Here's how the part is built. I have some questions about the finished solid (model axes, mm). A direction names the side the tool comes from. Round coordinates to 2 decimals unless told otherwise and drop trailing zeros. Loops run counter-clockwise (first coordinate to the right, second up) from the corner with the lowest first, then second, coordinate; pieces in that order, holes last. Notation, with made-up numbers: M 75,81.5 L 113,81.5 A24 ccw 113,115.5 Z; hole C 65.25,-34.5 d1. An arc over 180 degrees is marked long. Answer as CSV lines item,"result".
Autodesk Inventor part; units mm, degrees
ref_plane "YZ Plane" through (0, 0, 0) normal (1, 0, 0) x (0, 1, 0)
ref_plane "XZ Plane" through (0, 0, 0) normal (0, 1, 0) x (-1, 0, 0)
ref_plane "XY Plane" through (0, 0, 0) normal (0, 0, 1) x (1, 0, 0)
sketch "Sketch1" plane through (0, 0, 0) normal (0, 1, 0) x (-1, 0, 0)
  line L0 (27.5, -0.0615) -> (27.5, 89.9385)
  line L1 (-32.5, 89.9385) -> (-32.5, -0.0615)
  line L2 (-32.5, -0.0615) -> (-2.5, -0.0615)
  line L3 (-2.5, -0.0615) -> (-2.5, 89.9385) construction
  line L4 (-32.5, 44.9385) -> (-2.5, 44.9385) construction
  line L5 (-32.5, 89.9385) -> (27.5, 89.9385)
  line L6 (-21, 89.9385) -> (-9, 89.9385)
  line L7 (-9, 89.9385) -> (-9, 95.9385)
  line L8 (-9, 95.9385) -> (-21, 95.9385)
  line L9 (-21, 95.9385) -> (-21, 89.9385)
  line L10 (16, 89.9385) -> (4, 89.9385)
  line L11 (4, 89.9385) -> (4, 95.9385)
  line L12 (4, 95.9385) -> (16, 95.9385)
  line L13 (16, 95.9385) -> (16, 89.9385)
  line L14 (-2.5, 44.9385) -> (27.5, 44.9385) construction
  line L15 (-2.5, -0.0615) -> (27.5, -0.0615)
  line L16 (-9, 86.9385) -> (-21, 86.9385)
  line L17 (-21, 86.9385) -> (-21, 80.9385)
  line L18 (-21, 80.9385) -> (-9, 80.9385)
  line L19 (-9, 80.9385) -> (-9, 86.9385)
  line L20 (-9, 86.9385) -> (-21, 80.9385) construction
  line L21 (-21, 86.9385) -> (-9, 80.9385) construction
  line L22 (4, 86.9385) -> (16, 86.9385)
  line L23 (16, 86.9385) -> (16, 80.9385)
  line L24 (16, 80.9385) -> (4, 80.9385)
  line L25 (4, 80.9385) -> (4, 86.9385)
  line L26 (4, 86.9385) -> (16, 80.9385) construction
  line L27 (16, 86.9385) -> (4, 80.9385) construction
  point P0 (-15, 83.9385)
  point P1 (10, 83.9385)
  dimension "d0" = 60
  dimension "d1" = 90
  dimension "d18" = 12
  dimension "d19" = 6
  dimension "d20" = 18.5
  dimension "d21" = 12
  dimension "d22" = 6
  dimension "d23" = 3
extrude "Extrusion1" add sketch "Sketch1" along normal blind 6
sketch "Sketch2" plane through (0, 6, 0) normal (0, 1, 0) x (1, 0, 0)
  circle A0 centre (8, -19.9385) radius 1.4986
  circle A1 centre (27, -19.9385) radius 1.4986
  circle A2 centre (27, -36.4385) radius 1.4985
  circle A3 centre (8, -36.4385) radius 1.4985
  line L0 (27, -36.4385) -> (8, -36.4385) construction
  line L1 (8, -36.4385) -> (8, -19.9385) construction
  line L2 (8, -19.9385) -> (27, -19.9385) construction
  line L3 (27, -19.9385) -> (27, -36.4385) construction
  line L4 (27, -36.4385) -> (8, -19.9385) construction
  line L5 (27, -19.9385) -> (8, -36.4385) construction
  line L6 (32.5, 0.0615) -> (-27.5, 0.0615) construction
  line L7 (2.5, 0.0615) -> (2.5, -89.9385) construction
  line L8 (-4, -89.9385) -> (9, -89.9385) construction
  line L9 (-2.5, -49.9385) -> (-5.5, -49.9385)
  line L10 (-5.5, -49.9385) -> (-5.5, -43.9385)
  line L11 (-5.5, -43.9385) -> (-2.5, -43.9385)
  line L12 (-2.5, -43.9385) -> (-2.5, -49.9385)
  line L13 (-2.5, -28.9385) -> (-5.5, -28.9385)
  line L14 (-5.5, -28.9385) -> (-5.5, -22.9385)
  line L15 (-5.5, -22.9385) -> (-2.5, -22.9385)
  line L16 (-2.5, -22.9385) -> (-2.5, -28.9385)
  point P0 (0, 0)
  point P1 (17.5, -28.1885)
  dimension "d26" = 2.9972
  dimension "d28" = 2.9972
  dimension "d29" = 19
  dimension "d30" = 2.997
  dimension "d31" = 2.997
  dimension "d32" = 16.5
  dimension "d33" = 15
  dimension "d36" = 20
  dimension "d37" = 3
  dimension "d38" = 6
  dimension "d39" = 6
  dimension "d40" = 5
  dimension "d41" = 40
  dimension "d42" = 15
extrude "Extrusion2" cut sketch "Sketch2" against normal through all
properties part number "thumper-bumper-sidewall-v2"
1. If I drill on line 1 (Z direction, x = 27, y = 2.3); line 2 (X direction, y = 3.9, z = 26); line 3 (Z direction, x = -8, y = 4.4), over which ranges is the centre line in solid material (lowest first)? Write a range as [from, to].
Evaluation:
line 1,"z = [-0.06, 18.44], [21.44, 34.94], [37.94, 89.94]"
line 2,"x = [-27.5, -5.5], [-2.5, 32.5]"
line 3,"z = [-0.06, 80.94], [86.94, 95.94]"
2. We'd pull the mould along X, two halves only. Please class faces 1 (the flat face through (27, 3, 89.938)), 2 (the flat face through (-2.5, 3, 26)), 3 (the flat face through (32.5, 3, 46)), 4 (the flat face through (3, 3, 89.938)): pulls with the +X half, pulls with the -X half, needs draft (parallel to the pull), parting line crosses it, or undercut.
Evaluation:
face 1,"needs draft"
face 2,"undercut"
face 3,"pulls with the +X half"
face 4,"undercut"
3. I want a section at D-D, the plane y = 3.7. Count the separate pieces of the cut face and the enclosed holes in it, and give its area (3 significant figures).
Evaluation:
separate pieces,"1"
enclosed holes,"8"
area,"5,340 mm²"
4. Which directions (+Z, -Z, +X, -X, +Y, -Y) give clear straight access to the entire face, cutting with the end or side of a thin tool? Please do faces 5 (the flat face through (-16, 3, 84)), 6 (the flat face through (-27.5, 3, 44)), 7 (the flat face through (21, 3, 93)).
Evaluation:
face 5,"+Y, -Y"
face 6,"+Z, -Z, -X, +Y, -Y"
face 7,"+Z, +X, +Y, -Y"
5. I want a section at B-B, the plane z = 84. Please give me the cut outline in (x, y).
Evaluation:
outline,"M -27.5,0 L -16,0 L -16,6 L -27.5,6 Z; M -4,0 L 9,0 L 9,6 L -4,6 Z; M 21,0 L 32.5,0 L 32.5,6 L 21,6 Z"
6. I want a section at A-A, the plane z = 25. Please give me the cut outline in (x, y).
Evaluation:
outline,"M -27.5,0 L -5.5,0 L -5.5,6 L -27.5,6 Z; M -2.5,0 L 32.5,0 L 32.5,6 L -2.5,6 Z"
7. I want a section at C-C, the plane x = 8. Please give me the cut outline in (y, z).
Evaluation:
outline,"M 0,-0.06 L 6,-0.06 L 6,18.44 L 0,18.44 Z; M 0,21.44 L 6,21.44 L 6,34.94 L 0,34.94 Z; M 0,37.94 L 6,37.94 L 6,89.94 L 0,89.94 Z"
8. For P1, Ø2.5, axis at x = 27, z = 36.44, coming from the +Y side; P2, Ø1.8, axis at y = 3, z = 91.5, coming from the +X side; P3, Ø3.5, axis at x = 27, z = 19.94, coming from the +Y side; P4, Ø3, axis at y = 2.5, z = 93.5, coming from the -X side, each with a flat end and sliding along its axis, tell me the tip position at first contact or that it passes through.
Evaluation:
P1,"passes through"
P2,"stops at x = 21"
P3,"stops at y = 6"
P4,"stops at x = -16"
